```python
from build123d import *

# Parameters (mm, degrees)
SKETCH1_W           = 120
SKETCH1_H           = 120
SKETCH1_W_2         = 64.2
SKETCH1_H_2         = 58.2
BOSS_EXTRUDE1_DEPTH = 1
CHAMFER1_SIZE       = 0.5


with BuildPart() as part:
    # Sketch1 → Boss-Extrude1 (new body)
    with BuildSketch(Plane(origin=(0, 0, 0), x_dir=(1, 0, 0), z_dir=(0, 1, 0))):
        Rectangle(SKETCH1_W, SKETCH1_H)
        Rectangle(SKETCH1_W_2, SKETCH1_H_2, mode=Mode.SUBTRACT)
    extrude(amount=BOSS_EXTRUDE1_DEPTH)

    # Chamfer1
    chamfer1_edges = [part.edges().sort_by_distance(p)[0] for p in [
        (32.1, 1, 0),
        (0, 1, -29.1),
        (-32.1, 1, 0),
        (0, 1, 29.1),
    ]]
    chamfer(chamfer1_edges, length=CHAMFER1_SIZE)


solid = part.part
```
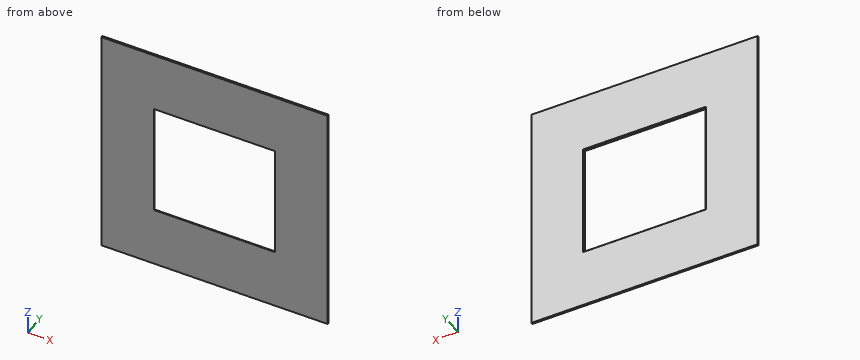
Geometry check sheet. Reference: the model listing, model coordinates, mm. Give positions to 0.01 mm unless a question says otherwise; leave off trailing zeros. Loops run counter-clockwise (first coordinate to the right, second up) from the corner with the lowest first, then second, coordinate; pieces in that order, holes last. Notation, with made-up numbers: M 5.5,-18.75 L 47.5,-18.75 A15 ccw 47.5,3.25 Z; hole C -21,57 d2. An arc over 180 degrees is marked long. Write item = value, one per line.
(1) Material ranges on line 1 (X direction, y = 0.3, z = 12); line 2 (Z direction, x = 27.5, y = 0.5); line 3 (Z direction, x = 14, y = 0.9), recorded low to high. Write a range as [from, to].
Answer below:
line_1 = [-60, -32.1], [32.1, 60]
line_2 = [-60, -29.1], [29.1, 60]
line_3 = [-60, -29.5], [29.5, 60]
(2) Sectioned sample at B-B, the plane x = -4. Record the cut outline in (y, z), plus the area to 4 significant figures.
Answer below:
outline = M 0,-60 L 1,-60 L 1,-29.6 L 0.5,-29.1 L 0,-29.1 Z; M 0,29.1 L 0.5,29.1 L 1,29.6 L 1,60 L 0,60 Z
area = 61.55 mm2
(3) Sectioned sample at A-A, the plane z = -8.5. Record the cut outline in (x, y), plus the area to 4 significant figures.
Answer below:
outline = M -60,0 L -32.1,0 L -32.1,0.5 L -32.6,1 L -60,1 Z; M 32.1,0 L 60,0 L 60,1 L 32.6,1 L 32.1,0.5 Z
area = 55.55 mm2
(4) Sectioned sample at C-C, the plane y = 0.75. Record the cut outline in (x, z), plus the area to 3 significant figures.
Answer below:
outline = M -60,-60 L 60,-60 L 60,60 L -60,60 Z; hole M -32.35,-29.35 L 32.35,-29.35 L 32.35,29.35 L -32.35,29.35 Z
area = 10,600 mm2
(5) Gauge pin test, flat end, axial feed: pin 1 Ø12 at (x, z) = (-27, 22.5) entering from -Y. Record the tip position at first contact, or that the pin passes through.
Answer below:
pin_1 = 0
